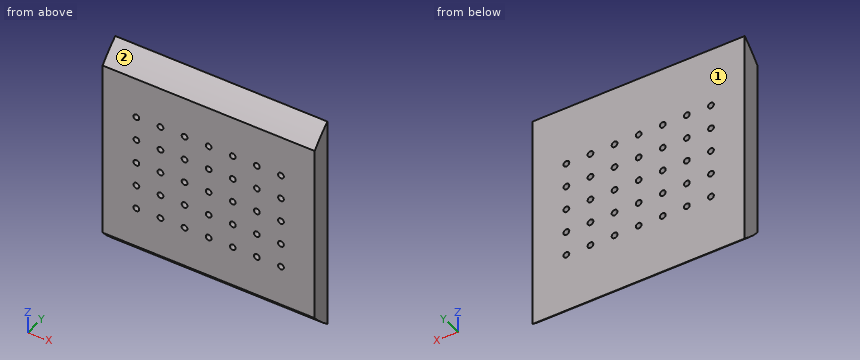
Autodesk Inventor part; units mm, degrees
ref_plane "YZ Plane" through (0, 0, 0) normal (1, 0, 0) x (0, 1, 0)
ref_plane "XZ Plane" through (0, 0, 0) normal (0, 1, 0) x (-1, 0, 0)
ref_plane "XY Plane" through (0, 0, 0) normal (0, 0, 1) x (1, 0, 0)
sketch "Sketch1" plane through (0, 0, 0) normal (1, 0, 0) x (0, 1, 0)
  circle A0 centre (0, 0) radius 71
  dimension "d0" = 142
extrude "Extrusion1" add sketch "Sketch1" along normal blind 110
sketch "Sketch2" plane through (110, 0, 0) normal (1, 0, 0) x (0, 0, -1)
  line L0 (0, 0) -> (0, -44.2)
  circle A0 centre (0, 0) radius 71
  line L1 (-55.564, -44.2) -> (55.564, -44.2)
  dimension "d3" = 44.2
extrude "Extrusion2" cut sketch "Sketch2" against normal blind 150 contours A0 L1 picked at (-0.2063, 32.437)
sketch "Sketch3" plane through (110, 0, 0) normal (1, 0, 0) x (0, 0, -1)
  line L0 (0, 0) -> (0, -54.2)
  arc A0 (-55.564, -44.2) -> (55.564, -44.2) centre (0, 0) ccw
  line L1 (-45.8624, -54.2) -> (45.8624, -54.2)
  dimension "d6" = 54.2
extrude "Extrusion3" cut sketch "Sketch3" against normal blind 150
sketch "Sketch7" plane through (110, -44.2, 55.564) normal (0, 1, 0) x (1, 0, 0)
  line L0 (-110, 0) -> (-110, 9.7016)
  line L1 (-110, 0) -> (-55, 0)
  line L2 (0, 0) -> (-110, 0)
  line L3 (-110, 111.128) -> (0, 111.128)
  line L4 (-55, 0) -> (-55, 55.64)
  circle A0 centre (-55, 55.64) radius 1.5
  point P0 (-110, 55.564)
  dimension "d71" = 55
  dimension "d72" = 111.128
  dimension "d73" = 55.64
  dimension "d75" = 3
extrude "Extrusion5" cut sketch "Sketch7" against normal blind 10
pattern_linear "Rectangular Pattern1" count 7 spacing 12.4968 along (-1, 0, 0) count 5 spacing 12.4968 along (0, 0, -1) of "Extrusion2", "Extrusion5" first direction both ways yes second direction both ways yes
properties part number "Base"
Could you check a few things on this model? Use its own coordinates, in mm. Face numbers are marked on the shaded views. Round coordinates to 2 decimals unless told otherwise and drop trailing zeros. Loops run counter-clockwise (first coordinate to the right, second up) from the corner with the lowest first, then second, coordinate; pieces in that order, holes last. Notation, with made-up numbers: (25.5, 24) -> (81.5, 24) arc R18 ccw to (81.5, 37) -> close; hole circle Ø5 at (73.5, 2.25). An arc over 180 degrees is marked (long way). Use CSV: the item, a comma, the result in double quotes.
(1) Suppose I cut it at C-C on x = 73. Write out the boundary of the cut face in (y, z), plus the area to 3 significant figures.
Return value:
outline,"(-54.2, -45.86) arc R71 ccw to (-44.2, -55.56) -> (-44.2, 55.56) arc R71 ccw to (-54.2, 45.86) -> close"
area,"1,020 mm²"
(2) Suppose I cut it at A-A on x = 55. Write out the boundary of the cut face in (y, z), plus the area to 3 significant figures.
Return value:
outline,"(-54.2, -45.86) arc R71 ccw to (-44.2, -55.56) -> (-44.2, -26.57) -> (-54.2, -26.57) -> close; (-54.2, -23.57) -> (-44.2, -23.57) -> (-44.2, -14.07) -> (-54.2, -14.07) -> close; (-54.2, -11.07) -> (-44.2, -11.07) -> (-44.2, -1.58) -> (-54.2, -1.58) -> close; (-54.2, 1.42) -> (-44.2, 1.42) -> (-44.2, 10.92) -> (-54.2, 10.92) -> close; (-54.2, 13.92) -> (-44.2, 13.92) -> (-44.2, 23.42) -> (-54.2, 23.42) -> close; (-54.2, 26.42) -> (-44.2, 26.42) -> (-44.2, 55.56) arc R71 ccw to (-54.2, 45.86) -> close"
area,"871 mm²"
(3) If I drill on probe 1 along Z at (x, y) = (55, -51.75); probe 2 along Z at (x, y) = (44.5, -48.75); probe 3 along Z at (x, y) = (74.5, -47.75), over which ranges is the centre line in solid material (lowest first)? Write a range as [from, to].
Return value:
probe 1,"z = [-48.61, -26.57], [-23.57, -14.07], [-11.07, -1.58], [1.42, 10.92], [13.92, 23.42], [26.42, 48.61]"
probe 2,"z = [-51.62, 51.62]"
probe 3,"z = [-52.54, 52.54]"
(4) Suppose I cut it at B-B on y = -51.5. Give the number of separate pieces and of enclosed holes in the cut face, plus the area to 3 significant figures.
Return value:
separate pieces,"1"
enclosed holes,"35"
area,"10,500 mm²"
(5) If we mould it in two halves opening along Z, with no side actions, what happens to the marked faces 1 and 2? For each: +Z half, -Z half, draft (parallel to the pull), parting line (faces both ways), or undercut.
Return value:
face 1,"draft"
face 2,"+Z half"
(6) Will these pins go through, and if not, where does the flat tip stop? pin 1 Ø1.8 at (x, z) = (55, -25.07) entering from -Y; pin 2 Ø3 at (x, y) = (45.5, -53) entering from -Z; pin 3 Ø6 at (x, y) = (67.5, -48) entering from +Z; pin 4 Ø6 at (x, y) = (31.5, -52.5) entering from -Z.
Return value:
pin 1,"passes through"
pin 2,"stops at z = -48.87"
pin 3,"stops at z = 54.92"
pin 4,"stops at z = -50.9"
